Input: part model. Units: mm. Frame: model coordinates. Face numbers are marked on the shaded views. A direction names the side the tool comes from. Coordinates: 2 decimals unless noted, no trailing zeros. Write each loop counter-clockwise with the first axis right and the second up, starting at its lowest first coordinate (ties: lowest second). Pieces come first, ordered by that corner, then holes. Notation, with made-up numbers: M 88,25 L 114,25 A19 cw 114,35 Z; hole C -20.75,-13.75 d8. An arc over 180 degrees is marked long. Write each question's results on one line, items separated by ' | '. Start each with the question number.
1. Ray query, probe 1 along Y at (x, z) = (0, 1); probe 2 along Y at (x, z) = (-2, -8); probe 3 along Z at (x, y) = (-1, 17). Return the intervals inside material, ascending.
2. Section query B-B, the plane z = 0. Output: boundary loops of the cut face in (x, y), and give its area (3 significant figures).
3. Pull-direction query (Y, two-part tool) for the marked faces 4, 5 and 6; classes: +Y half, -Y half, draft (parallel to the pull), parting line (faces both ways), or undercut.
4. Section query A-A, the plane x = 0. Output: boundary loops of the cut face in (y, z).
5. Set-up query: the marked faces 1, 2 and 3. Return all of +Z, -Z, +X, -X, +Y, -Y with unobstructed straight access to the full face (end or side cutting, diameter ignored); none if empty.
6. First-contact query: pin 1 (8 mm diameter, centred on x = 6.5, y = 11, fed in from +Z); pin 2 (8 mm diameter, centred on x = 10.5, y = 3.5, fed in from -Z); pin 3 (1.5 mm diameter, centred on x = -2.5, y = 12.5, fed in from +Z). Flat tips, straight axial feed; report the tip coordinate or a pass-through.
7. Section query C-C, the plane y = 11.75. Output: boundary loops of the cut face in (x, z) (1 decimal).
8. Section query D-D, the plane y = 5.5. Output: boundary loops of the cut face in (x, z), and give its area (3 significant figures).
Autodesk Inventor part; units mm, degrees
ref_plane "Work Plane1" through (0, 9.9822, -4.7625) normal (0, 0, 1) x (1, 0, 0)
ref_plane "YZ Plane" through (0, 0, 0) normal (1, 0, 0) x (0, 1, 0)
ref_plane "XZ Plane" through (0, 0, 0) normal (0, 1, 0) x (-1, 0, 0)
sketch "Sketch1" plane through (0, 0, 0) normal (0, 1, 0) x (-1, 0, 0)
  circle A0 centre (0, 0) radius 15.7353
  dimension "d0" = 31.4706
extrude "Extrusion1" add sketch "Sketch1" along normal blind 2.54
sketch "Sketch2" plane through (0, 2.54, 0) normal (0, 1, 0) x (1, 0, 0)
  circle A0 centre (0, 0) radius 12.6365
  dimension "d3" = 25.273
extrude "Extrusion2" add sketch "Sketch2" along normal blind 4.9022
sketch "Sketch3" plane through (0, 7.4422, 0) normal (0, 1, 0) x (1, 0, 0)
  circle A0 centre (0, 0) radius 15.7353
  dimension "d6" = 31.4706
extrude "Extrusion3" add sketch "Sketch3" along normal blind 2.54
chamfer "Chamfer1" distance 1.27 angle 45 2 edges at (-15.7353, 9.9822, 0) (15.7353, 0, 0)
sketch "Sketch4" plane through (0, 9.9822, 0) normal (0, 1, 0) x (1, 0, 0)
  circle A0 centre (0, 0) radius 4.7625
  dimension "d12" = 9.525
extrude "Extrusion4" add sketch "Sketch4" along normal blind 9.525
ref_plane "Work Plane1" through (0, 9.9822, -4.7625) normal (0, 0, 1) x (1, 0, 0)
sketch "Sketch5" plane through (0, 9.9822, -4.7625) normal (0, 0, 1) x (1, 0, 0)
  circle A0 centre (0, 4.7625) radius 1.7526
  line L0 (-14.4653, 0) -> (14.4653, 0)
  point P0 (0, -9.9822)
  dimension "d15" = 3.5052
  dimension "d16" = 4.7625
extrude "Extrusion5" cut sketch "Sketch5" along normal blind 9.525
properties part number "Plug" material "Acetal Resin, Black"
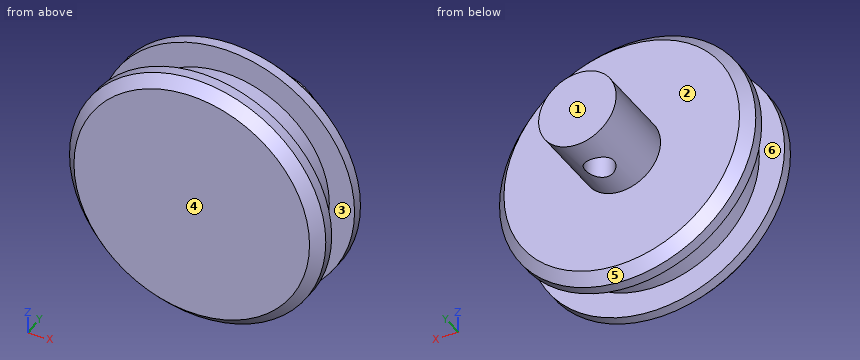
Answer:
1) probe 1: 0 to 12.99, 16.5 to 19.51 | probe 2: 0 to 9.98 | probe 3: -4.66 to 4.66
2) outline: M -15.74,1.27 L -14.47,0 L 14.47,0 L 15.74,1.27 L 15.74,2.54 L 12.64,2.54 L 12.64,7.44 L 15.74,7.44 L 15.74,8.71 L 14.47,9.98 L 4.76,9.98 L 4.76,19.51 L -4.76,19.51 L -4.76,9.98 L -14.47,9.98 L -15.74,8.71 L -15.74,7.44 L -12.64,7.44 L -12.64,2.54 L -15.74,2.54 Z; hole C 0,14.74 d3.51 | area: 362 mm^2
3) face 4: -Y half | face 5: +Y half | face 6: undercut
4) outline: M 0,-14.47 L 1.27,-15.74 L 2.54,-15.74 L 2.54,-12.64 L 7.44,-12.64 L 7.44,-15.74 L 8.71,-15.74 L 9.98,-14.47 L 9.98,-4.76 L 12.99,-4.76 L 12.99,4.76 L 9.98,4.76 L 9.98,14.47 L 8.71,15.74 L 7.44,15.74 L 7.44,12.64 L 2.54,12.64 L 2.54,15.74 L 1.27,15.74 L 0,14.47 Z; M 16.5,-4.76 L 19.51,-4.76 L 19.51,4.76 L 16.5,4.76 Z
5) face 1: +Z, -Z, +X, -X, +Y | face 2: +Y | face 3: none
6) pin 1: z = 15.4 | pin 2: z = -14.28 | pin 3: z = 4.43
7) outline: C 0,0 d9.5
8) outline: C 0,0 d25.27 | area: 502 mm^2
